For this review, take the finished solid that the model builds, in its own axes (mm). A direction names the side the tool comes from. Round coordinates to 2 decimals unless told otherwise and drop trailing zeros. Order: outer loops, then holes, each group sorted by start corner. A loop starts at its lowest first (then second) coordinate and runs counter-clockwise, first axis right, second up. Notation, with made-up numbers: M 58.5,-38.5 L 105.5,-38.5 A29 ccw 105.5,-12.5 Z; hole C 76.25,49.5 d1. An arc over 180 degrees is marked long. Put each result on its own line as item: value.
from build123d import *

# Parameters (mm, degrees)
F3_R     = 5
F2_R     = 5.970873
F4_DEPTH = 25


with BuildPart() as f1:
    # F0 (on Front) → F1 (revolve)
    with BuildSketch(Plane.XZ):
        Polygon((7.159092, 15.552509), (0, 15.552509), (0, 8.146551), (22.464735, 8.146551), (22.464735, 15.552509), (12.836992, 15.552509), (12.836992, 36.289185), (28.636364, 36.289185), (28.636364, 44.188876), (0, 44.188876), (0, 36.289185), (7.159092, 36.289185), align=None)
    revolve(axis=Axis((9.257446, 0, 0), (1, 0, 0)))

    # F3
    f3_edges = [f1.edges().sort_by_distance(p)[0] for p in [
        (28.636364, 0, -44.188876),
        (0, 0, -44.188876),
    ]]
    fillet(f3_edges, radius=F3_R)

    # F2 (on face) → F4 (cut)
    with BuildSketch(Plane(origin=(7.159092, 0, 0), x_dir=(0, -1, 0), z_dir=(-1, 0, 0))):
        with Locations((0, 26.167713)):
            Circle(F2_R)
        with Locations((-24.886974, 8.086268)):
            Circle(F2_R)
        with Locations((24.886974, 8.086268)):
            Circle(F2_R)
        with Locations((-15.380996, -21.170125)):
            Circle(F2_R)
        with Locations((15.380996, -21.170125)):
            Circle(F2_R)
    extrude(amount=-F4_DEPTH, mode=Mode.SUBTRACT)


solid = f1.part
(1) Add section C-C on y = 0. State how many separate pieces and enclosed holes the cut face has, then the cut area to 3 significant figures.
A:
separate pieces: 3
enclosed holes: 0
area: 931 mm2
(2) For faces 1 (the face through (20.847, 35.426, -7.867)), 2 (the face through (3.63, 35.426, -7.867)), 3 (the face through (10, -14.1, -27)), list the 3-axis set-ups (+Z, -Z, +X, -X, +Y, -Y) from which the entire face can be reached by the end or side of a thin tool; tool diameter is ignored.
A:
face 1: +X
face 2: -X
face 3: +X, -X
(3) Draft analysis for pull direction Z (two halves, no side actions). For faces 4 (the face through (0, 35, 11)), 5 (the face through (12.837, 16, 1)), 6 (the face through (14.188, 43.138, -9.579)), state which applies: released by +Z, released by -Z, zero draft, split by the parting line, or undercut.
A:
face 4: zero draft
face 5: undercut
face 6: split by the parting line
(4) Add section A-A on z = 0. Give the boundary of the cut face in (x, y), then the cut area to 3 significant figures.
A:
outline: M 0,-39.19 A5 ccw 5,-44.19 L 23.64,-44.19 A5 ccw 28.64,-39.19 L 28.64,-36.29 L 12.84,-36.29 L 12.84,-15.55 L 22.46,-15.55 L 22.46,-8.15 L 0,-8.15 L 0,-15.55 L 7.16,-15.55 L 7.16,-36.29 L 0,-36.29 Z; M 0,8.15 L 22.46,8.15 L 22.46,15.55 L 12.84,15.55 L 12.84,36.29 L 28.64,36.29 L 28.64,39.19 A5 ccw 23.64,44.19 L 5,44.19 A5 ccw 0,39.19 L 0,36.29 L 7.16,36.29 L 7.16,15.55 L 0,15.55 Z
area: 999 mm2
(5) Add section B-B on x = 16.75. Give the boundary of the cut face in (y, z).
A:
outline: C 0,0 d88.38; C 0,0 d31.11; hole C 0,0 d72.58; hole C 0,0 d16.29
(6) To check wall thickness, follow L1, parallel to Y at x = 17.25, z = 0; L2, parallel to Z at x = 18.5, y = -9; L3, parallel to X at y = 1.5, z = 10. State the ranges of each line that lie inside material, in increasing order.
A:
L1: y = -44.19 to -36.29, -15.55 to -8.15, 8.15 to 15.55, 36.29 to 44.19
L2: z = -43.26 to -35.16, -12.68 to 12.68, 35.16 to 43.26
L3: x = 0 to 22.46
(7) Insertion check: pin 1 Ø13.5 at (y, z) = (15.38, -21.17) entering from -X; pin 2 Ø10 at (x, y) = (20, -10) entering from -Z; pin 3 Ø25 at (y, z) = (4.5, 0.5) entering from +X. Each pin has a flat end and moves straight along its axis. Give the tip position at first contact, or say it passes through.
A:
pin 1: stops at x = 7.16
pin 2: stops at z = -43.91
pin 3: stops at x = 22.46
